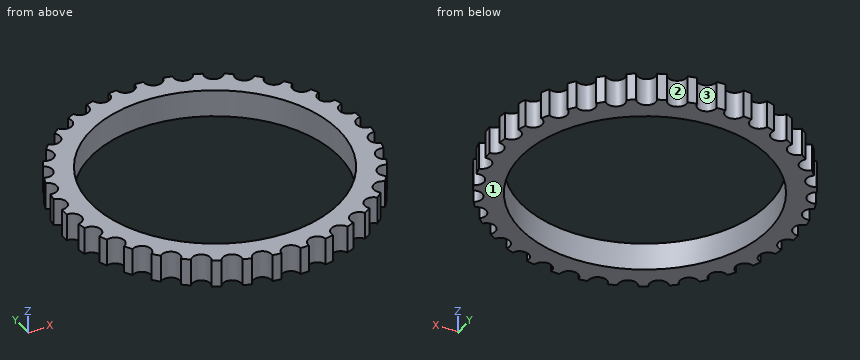
```python
from build123d import *

# Parameters (mm, degrees)
SKETCH1_R           = 27.852115
SKETCH1_R_2         = 22.852115
BOSS_EXTRUDE1_DEPTH = 5
SKETCH3_R           = 1.7
CUT_EXTRUDE1_DEPTH  = 8


with BuildPart() as part:
    # Sketch1 → Boss-Extrude1 (new body)
    with BuildSketch(Plane.XY):
        Circle(SKETCH1_R)
        Circle(SKETCH1_R_2, mode=Mode.SUBTRACT)
    extrude(amount=BOSS_EXTRUDE1_DEPTH)

    # Sketch3 → Cut-Extrude1 (cut, symmetric)
    with BuildSketch(Plane.XY.offset(2.5)):
        with Locations((27.852115, 0)):
            Circle(SKETCH3_R)
        with Locations((27.404520054, -4.973187168)):
            Circle(SKETCH3_R)
        with Locations((26.076121284, -9.786532008)):
            Circle(SKETCH3_R)
        with Locations((23.909614521, -14.285329658)):
            Circle(SKETCH3_R)
        with Locations((20.974633074, -18.324985058)):
            Circle(SKETCH3_R)
        with Locations((17.365509663, -21.77566036)):
            Circle(SKETCH3_R)
        with Locations((13.198244482, -24.526448022)):
            Circle(SKETCH3_R)
        with Locations((8.606776864, -26.488935463)):
            Circle(SKETCH3_R)
        with Locations((3.738680356, -27.600046724)):
            Circle(SKETCH3_R)
        with Locations((-1.249580414, -27.824069774)):
            Circle(SKETCH3_R)
        with Locations((-6.197678642, -27.153804327)):
            Circle(SKETCH3_R)
        with Locations((-10.94657838, -25.610793267)):
            Circle(SKETCH3_R)
        with Locations((-15.343646081, -23.244630239)):
            Circle(SKETCH3_R)
        with Locations((-19.247556372, -20.131365669)):
            Circle(SKETCH3_R)
        with Locations((-22.532834364, -16.371062442)):
            Circle(SKETCH3_R)
        with Locations((-25.09388852, -12.084579799)):
            Circle(SKETCH3_R)
        with Locations((-26.848404452, -7.409688817)):
            Circle(SKETCH3_R)
        with Locations((-27.739990573, -2.49664434)):
            Circle(SKETCH3_R)
        with Locations((-27.739990573, 2.49664434)):
            Circle(SKETCH3_R)
        with Locations((-26.848404452, 7.409688817)):
            Circle(SKETCH3_R)
        with Locations((-25.09388852, 12.084579799)):
            Circle(SKETCH3_R)
        with Locations((-22.532834364, 16.371062442)):
            Circle(SKETCH3_R)
        with Locations((-19.247556372, 20.131365669)):
            Circle(SKETCH3_R)
        with Locations((-15.343646081, 23.244630239)):
            Circle(SKETCH3_R)
        with Locations((-10.94657838, 25.610793267)):
            Circle(SKETCH3_R)
        with Locations((-6.197678642, 27.153804327)):
            Circle(SKETCH3_R)
        with Locations((-1.249580414, 27.824069774)):
            Circle(SKETCH3_R)
        with Locations((3.738680356, 27.600046724)):
            Circle(SKETCH3_R)
        with Locations((8.606776864, 26.488935463)):
            Circle(SKETCH3_R)
        with Locations((13.198244482, 24.526448022)):
            Circle(SKETCH3_R)
        with Locations((17.365509663, 21.77566036)):
            Circle(SKETCH3_R)
        with Locations((20.974633074, 18.324985058)):
            Circle(SKETCH3_R)
        with Locations((23.909614521, 14.285329658)):
            Circle(SKETCH3_R)
        with Locations((26.076121284, 9.786532008)):
            Circle(SKETCH3_R)
        with Locations((27.404520054, 4.973187168)):
            Circle(SKETCH3_R)
    extrude(amount=CUT_EXTRUDE1_DEPTH, both=True, mode=Mode.SUBTRACT)


solid = part.part
```
The listing builds one solid part. Answer for the finished solid, in the listing's coordinates (mm). Face numbers are marked on the shaded views. Coordinates: 2 decimals unless noted, no trailing zeros. Write each loop counter-clockwise with the first axis right and the second up, starting at its lowest first coordinate (ties: lowest second). Pieces come first, ordered by that corner, then holes. Notation, with made-up numbers: M 40.5,48.25 L 77.5,48.25 A21 cw 77.5,55.25 Z; hole C 69.25,34.25 d8. An arc over 180 degrees is marked long. Use a Markdown table: item, result. Add a question column.
1. For a pull along X with two mould halves and no side action, classify the marked faces 1, 2 and 3 as +X half, -X half, draft (parallel to the pull), parting line (faces both ways), or undercut.
2. Section B-B (x = -1.5) is taken. Give the vertices of the cut face in (y, z).
3. Section A-A (y = 0) is taken. Give the vertices of the cut face in (x, z), plus the area to 3 significant figures.
4. Given P1, Ø1.5, axis at y = 19.5, z = 4.5, coming from the +X side; P2, Ø1, axis at x = -14.5, z = 2, coming from the +Y side, each flat-ended and moving along its own axis, determine where each tip first touches the part or whether it passes through.
5. Straight lines are drawn through the part: line 1 along Y through (x, z) = (1, 4.8); line 2 along Y through (x, z) = (0, 2.95); line 3 along X through (y, z) = (10, 0.75) (3 decimals). For each, find the intervals that lie inside material, in ascending order. Write a range as [from, to].
Data:
| question | item | result |
|---|---|---|
| 1 | face 1 | draft |
| 1 | face 2 | undercut |
| 1 | face 3 | undercut |
| 2 | outline | M -26.14,0 L -22.8,0 L -22.8,5 L -26.14,5 Z; M 22.8,0 L 26.14,0 L 26.14,5 L 22.8,5 Z |
| 3 | outline | M -27.85,0 L -22.85,0 L -22.85,5 L -27.85,5 Z; M 22.85,0 L 26.15,0 L 26.15,5 L 22.85,5 Z |
| 3 | area | 41.5 mm2 |
| 4 | P1 | stops at x = 19.82 |
| 4 | P2 | stops at y = 22.2 |
| 5 | line 1 | y = [-27.83, -22.83], [22.83, 27.83] |
| 5 | line 2 | y = [-26.67, -22.85], [22.85, 26.67] |
| 5 | line 3 | x = [-25.995, -20.548], [20.548, 24.39] |
